```python
from build123d import *

# Parameters (mm, degrees)
SKETCH1_R           = 1.999999997
SKETCH1_R_2         = 10.999999998
SKETCH1_R_3         = 1.999999998
BOSS_EXTRUDE1_DEPTH = 6


with BuildPart() as part:
    # Sketch1 → Boss-Extrude1 (new body)
    with BuildSketch(Plane.XY):
        with BuildLine():
            Line((-57.700744027, 162.345498824), (-95.228511524, 162.345498823))
            ThreePointArc((-95.228511524, 162.345498823), (-100.228511524, 161.005752861), (-103.888765562, 157.345498823))
            Line((-103.888765562, 157.345498823), (-122.65264931, 124.845498823))
            ThreePointArc((-122.65264931, 124.845498823), (-123.992395272, 119.845498822), (-122.65264931, 114.845498822))
            Line((-122.65264931, 114.845498822), (-103.88876556, 82.345498823))
            ThreePointArc((-103.88876556, 82.345498823), (-100.228511522, 78.685244785), (-95.228511522, 77.345498823))
            Line((-95.228511522, 77.345498823), (-73.987721784, 77.345498823))
            Line((-73.987721784, 77.345498823), (-73.987721784, 81.491705925))
            ThreePointArc((-73.987721784, 81.491705925), (-73.317848803, 83.991705925), (-71.487721784, 85.821832944))
            Line((-71.487721784, 85.821832944), (-49.487721784, 98.523538865))
            ThreePointArc((-49.487721784, 98.523538865), (-46.987721783, 99.193411846), (-44.487721784, 98.523538865))
            Line((-44.487721784, 98.523538865), (-40.897001108, 96.450435316))
            Line((-40.897001108, 96.450435316), (-30.276606238, 114.845498825))
            ThreePointArc((-30.276606238, 114.845498825), (-28.936860276, 119.845498825), (-30.276606239, 124.845498826))
            Line((-30.276606239, 124.845498826), (-49.040489989, 157.345498825))
            ThreePointArc((-49.040489989, 157.345498825), (-52.700744027, 161.005752862), (-57.700744027, 162.345498824))
        make_face()
        with Locations((-38.936860277, 119.845498824)):
            Circle(SKETCH1_R, mode=Mode.SUBTRACT)
        with Locations((-95.228511522, 87.345498823)):
            Circle(SKETCH1_R, mode=Mode.SUBTRACT)
        with Locations((-76.464627774, 119.845498824)):
            Circle(SKETCH1_R_2, mode=Mode.SUBTRACT)
        with Locations((-95.228511523, 152.345498823)):
            Circle(SKETCH1_R_3, mode=Mode.SUBTRACT)
    extrude(amount=BOSS_EXTRUDE1_DEPTH)


solid = part.part
```
Build history of the part. All positions in model axes, mm. A direction names the side the tool comes from. Give positions to 0.01 mm unless a question says otherwise; leave off trailing zeros. Loops run counter-clockwise (first coordinate to the right, second up) from the corner with the lowest first, then second, coordinate; pieces in that order, holes last.
Item 1: Flat gauge pins, fed straight in: pin 1 (1.5 mm diameter, centred on y = 151, z = 1.5, fed in from +X); pin 2 (1.2 mm diameter, centred on y = 80, z = 3, fed in from +X); pin 3 (2 mm diameter, centred on y = 116, z = 2, fed in from +X). Where does each tip first touch, or does it go through?
Answers follow:
pin 1: stops at x = -44.94
pin 2: stops at x = -73.99
pin 3: stops at x = -29.35
Item 2: Slice it at D-D, the plane x = -105.5. List the corners of the cut face in (y, z).
Answers follow:
outline: (85.14, 0) - (154.55, 0) - (154.55, 6) - (85.14, 6) - close
Item 3: Slice it at B-B, the plane x = -39.5. List the corners of the cut face in (y, z), and give its area (3 significant figures).
Answers follow:
outline: (98.87, 0) - (117.93, 0) - (117.93, 6) - (98.87, 6) - close; (121.76, 0) - (140.82, 0) - (140.82, 6) - (121.76, 6) - close
area: 229 mm2
Item 4: Slice it at C-C, the plane y = 94.5. List the corners of the cut face in (x, z).
Answers follow:
outline: (-110.91, 0) - (-56.46, 0) - (-56.46, 6) - (-110.91, 6) - close
Item 5: Drill centre lines: line 1 (X direction, y = 116, z = 1.05); line 2 (X direction, y = 126.5, z = 4); line 3 (Y direction, x = -74.5, z = 3.3). Where is each one in solid material? Low to high.
Answers follow:
line 1: x = -123.22 to -86.77, -66.16 to -29.71
line 2: x = -121.7 to -85.22, -67.71 to -31.23
line 3: y = 77.35 to 109.02, 130.67 to 162.35
Item 6: Which spindle directions (+Z, -Z, +X, -X, +Y, -Y) get a long thin tool onto all of the face, cutting with end or side? Do faces 1 (the face through (-73.988, 79, 3)), 2 (the face through (-87.454, 120.329, 2.958)), 3 (the face through (-42.717, 97.501, 2.958)). Say none if no direction does.
Answers follow:
face 1: +Z, -Z, +X, -Y
face 2: +Z, -Z
face 3: +Z, -Z, -Y
Item 7: Slice it at A-A, the plane z = 2.15. List the corners of the cut face in (x, y), and give its area (3 significant figures).
Answers follow:
outline: (-122.65, 114.85) - (-103.89, 82.35) arc R10 ccw to (-95.23, 77.35) - (-73.99, 77.35) - (-73.99, 81.49) arc R5 cw to (-71.49, 85.82) - (-49.49, 98.52) arc R5 cw to (-44.49, 98.52) - (-40.9, 96.45) - (-30.28, 114.85) arc R10 ccw to (-30.28, 124.85) - (-49.04, 157.35) arc R10 ccw to (-57.7, 162.35) - (-95.23, 162.35) arc R10 ccw to (-103.89, 157.35) - (-122.65, 124.85) arc R10 ccw to start; hole circle Ø4 at (-95.23, 87.35); hole circle Ø4 at (-95.23, 152.35); hole circle Ø22 at (-76.46, 119.85); hole circle Ø4 at (-38.94, 119.85)
area: 5,390 mm2
